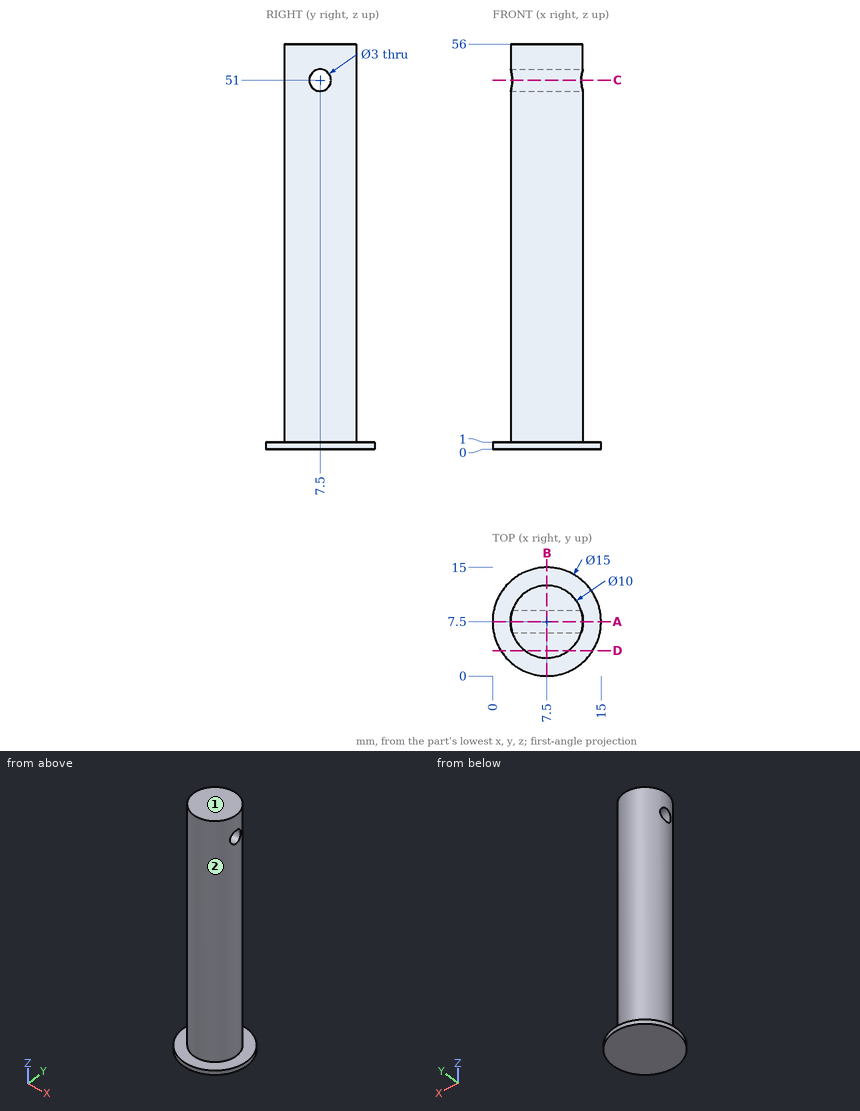
Print and shaded views of the part. All mm, measured from the part's lowest x, y and z. A direction names the side the tool comes from. Coordinates: 2 decimals unless noted, no trailing zeros. Order: outer loops, then holes, each group sorted by start corner. A loop starts at its lowest first (then second) coordinate and runs counter-clockwise, first axis right, second up. Notation, with made-up numbers: (-23, 53.5) - (20, 53.5) arc R18 ccw to (20, 86.5) - close; hole circle Ø11 at (58.5, 44). An arc over 180 degrees is marked (long way). Return JSON: item names as keys, results as strings. Group by question number.
Item 1: Cut at C-C (z = 51). List the corners of the cut face in (x, y).
Item 2: Cut at A-A (y = 7.5). List the corners of the cut face in (x, z), plus the area to 3 significant figures.
Item 3: Cut at B-B (x = 7.5). List the corners of the cut face in (y, z), plus the area to 3 significant figures.
Item 4: Pin check, flat tips, straight feed: pin 1 (8 mm diameter, centred on x = 6.5, z = 46, fed in from -Y); pin 2 (1.5 mm diameter, centred on x = 12, z = 17, fed in from -Y); pin 3 (1.8 mm diameter, centred on y = 7.5, z = 51, fed in from +X); pin 4 (2 mm diameter, centred on y = 6, z = 45, fed in from +X). Stop position of each tip, or through.
Item 5: Drill centre lines: probe 1 along Z at (x, y) = (8.5, 7.5); probe 2 along Z at (x, y) = (2.5, 12.75); probe 3 along Y at (x, z) = (7.75, 51). Where is each one in solid material? Low to high. Write a range as from..to.
Item 6: Which spindle directions (+Z, -Z, +X, -X, +Y, -Y) get a long thin tool onto all of the face, cutting with end or side? Do the marked faces 1 and 2. Say none if no direction does.
Item 7: Cut at D-D (y = 3.5). List the corners of the cut face in (x, z), plus the area to 3 significant figures.
Check values:
{
 "1": {"outline": "(2.73, 6) arc R5 ccw to (12.27, 6) - close; (2.73, 9) - (12.27, 9) arc R5 ccw to start"},
 "2": {"outline": "(0, 0) - (15, 0) - (15, 1) - (12.5, 1) - (12.5, 49.5) - (2.5, 49.5) - (2.5, 1) - (0, 1) - close; (2.5, 52.5) - (12.5, 52.5) - (12.5, 56) - (2.5, 56) - close", "area": "535 mm2"},
 "3": {"outline": "(0, 0) - (15, 0) - (15, 1) - (12.5, 1) - (12.5, 56) - (2.5, 56) - (2.5, 1) - (0, 1) - close; hole circle Ø3 at (7.5, 51)", "area": "558 mm2"},
 "4": {"pin 1": "stops at y = 2.5", "pin 2": "stops at y = 4.19", "pin 3": "passes through", "pin 4": "stops at x = 12.47"},
 "5": {"probe 1": "z = 0..49.5, 52.5..56", "probe 2": "z = 0..1", "probe 3": "y = 2.51..6, 9..12.49"},
 "6": {"face 1": "+Z, +X, -X, +Y, -Y", "face 2": "+Z"},
 "7": {"outline": "(1.16, 0) - (13.84, 0) - (13.84, 1) - (10.5, 1) - (10.5, 56) - (4.5, 56) - (4.5, 1) - (1.16, 1) - close", "area": "343 mm2"}
}
